Work out the finished part from the listing and answer in its coordinate system (mm). A direction names the side the tool comes from. Give positions to 0.01 mm unless a question says otherwise; leave off trailing zeros. Loops run counter-clockwise (first coordinate to the right, second up) from the corner with the lowest first, then second, coordinate; pieces in that order, holes last. Notation, with made-up numbers: (47, -0.75) - (75, -0.75) arc R29 ccw to (75, 36.25) - close; hole circle Ø9 at (-18, 12). An arc over 180 degrees is marked (long way). One line per question, with ' | ' between items.
from build123d import *

# Parameters (mm, degrees)
SKETCH2_W                = 211.751333334
SKETCH2_H                = 164
BOSS_EXTRUDE1_DEPTH      = 74.083333333
CUT_EXTRUDE7_DEPTH       = 70.90833333
CUT_EXTRUDE9_REACH       = 240.853
CUT_EXTRUDE10_DEPTH      = 3.175
SKETCH14_W               = 205.401333334
SKETCH14_H               = 3.175
CUT_EXTRUDE11_DEPTH      = 3.175
CUT_EXTRUDE12_DEPTH      = 239.853443446
CUT_EXTRUDE12_DEPTH_BACK = 3.175
CUT_EXTRUDE14_REACH      = 210.792
SKETCH18_R               = 3.025
LPATTERN2_COUNT          = 4
LPATTERN2_PITCH          = 46.99
CUT_EXTRUDE15_REACH      = 210.792
SKETCH19_R               = 3.025
LPATTERN3_COUNT          = 4
LPATTERN3_PITCH          = 46.99
BOSS_EXTRUDE2_DEPTH      = 70.866
SKETCH25_W               = 3.175
SKETCH25_H               = 19.00766667
BOSS_EXTRUDE3_DEPTH      = 3.175
CUT_EXTRUDE18_REACH      = 211.317
CUT_EXTRUDE19_REACH      = 155.042
SKETCH16_R               = 3.025
CUT_EXTRUDE20_DEPTH      = 210.317467246
LPATTERN4_COUNT          = 3
LPATTERN4_PITCH          = 50.8
SKETCH20_R               = 3.025
CUT_EXTRUDE21_DEPTH      = 210.317467246


with BuildPart() as part:
    # Sketch2 → Boss-Extrude1 (new body)
    with BuildSketch(Plane.XY):
        Rectangle(SKETCH2_W, SKETCH2_H)
    extrude(amount=BOSS_EXTRUDE1_DEPTH)

    # Sketch9 → Cut-Extrude7 (cut)
    with BuildSketch(Plane.XY.offset(74.083333333)):
        Polygon((-102.700666667, 62.95), (-102.700666667, -47.748173381), (-102.700666667, -78.825), (-61.266487403, -78.825), (102.700666667, -78.825), (102.700666667, -21.962957065), (102.700666667, 78.825), (-87.76182231, 78.825), (-102.700666667, 78.825), align=None)
    extrude(amount=-CUT_EXTRUDE7_DEPTH, mode=Mode.SUBTRACT)

    # Sketch11 → Cut-Extrude9 (cut, up to next)
    with BuildSketch(Plane.ZY.offset(105.875666667), mode=Mode.PRIVATE) as cut_extrude9_sk1:
        Polygon((58.208333333, 78.825), (74.083333333, 62.95), (74.083333333, 82), (58.208333333, 82), (58.208333333, 79.62382388), align=None)
    cut_extrude9_tool1 = extrude(cut_extrude9_sk1.sketch, amount=-CUT_EXTRUDE9_REACH, mode=Mode.PRIVATE) & part.part
    add(cut_extrude9_tool1.solids().sort_by_distance((-105.875667, 75.49881, 68.035714))[0], mode=Mode.SUBTRACT)

    # Sketch13 → Cut-Extrude10 (cut)
    with BuildSketch(Plane.ZY.offset(105.875666667)):
        Polygon((58.208333333, 78.825), (55.033333333, 82), (58.208333333, 82), align=None)
    extrude(amount=-CUT_EXTRUDE10_DEPTH, mode=Mode.SUBTRACT)

    # Sketch14 → Cut-Extrude11 (cut)
    with BuildSketch(Plane.XY.offset(58.208333333)):
        with Locations((0, 80.4125)):
            Rectangle(SKETCH14_W, SKETCH14_H)
    extrude(amount=-CUT_EXTRUDE11_DEPTH, mode=Mode.SUBTRACT)

    # Sketch15 → Cut-Extrude12 (cut, two sides: drawn at the far end of the back side and taken through both)
    with BuildSketch(Plane(origin=(105.875666667, 0, 0), x_dir=(0, 0, -1), z_dir=(1, 0, 0)).offset(-CUT_EXTRUDE12_DEPTH_BACK)):
        Polygon((-58.208333333, 79.215720039), (-58.208333333, 78.825), (-55.033333333, 82), (-58.208333333, 82), align=None)
    extrude(amount=CUT_EXTRUDE12_DEPTH + CUT_EXTRUDE12_DEPTH_BACK, mode=Mode.SUBTRACT)

    # Sketch18 → Cut-Extrude14 (cut, up to next)
    with BuildSketch(Plane.XZ.offset(82), mode=Mode.PRIVATE) as cut_extrude14_sk1:
        with Locations(Location((-89.365666667, 66.463333333, 0), (0, 0, 270))):
            Circle(SKETCH18_R)
    cut_extrude14_tool1 = extrude(cut_extrude14_sk1.sketch, amount=-CUT_EXTRUDE14_REACH, mode=Mode.PRIVATE) & part.part
    cut_extrude14 = cut_extrude14_tool1.solids().sort_by_distance((-89.365667, -82, 66.463333))[0]
    add(cut_extrude14, mode=Mode.SUBTRACT)

    # LPattern2: Cut-Extrude14 ×4
    with Locations(*[(i * LPATTERN2_PITCH, 0, 0) for i in range(1, LPATTERN2_COUNT)]):
        add(cut_extrude14, mode=Mode.SUBTRACT)

    # Sketch19 → Cut-Extrude15 (cut, up to next)
    with BuildSketch(Plane(origin=(0, 82, 0), x_dir=(1, 0, 0), z_dir=(0, 1, 0)), mode=Mode.PRIVATE) as cut_extrude15_sk1:
        with Locations(Location((-88.125666667, -48.683333333, 0), (0, 0, 270))):
            Circle(SKETCH19_R)
    cut_extrude15_tool1 = extrude(cut_extrude15_sk1.sketch, amount=-CUT_EXTRUDE15_REACH, mode=Mode.PRIVATE) & part.part
    cut_extrude15 = cut_extrude15_tool1.solids().sort_by_distance((-88.125667, 82, 48.683333))[0]
    add(cut_extrude15, mode=Mode.SUBTRACT)

    # LPattern3: Cut-Extrude15 ×4
    with Locations(*[(i * LPATTERN3_PITCH, 0, 0) for i in range(1, LPATTERN3_COUNT)]):
        add(cut_extrude15, mode=Mode.SUBTRACT)

    # Sketch22 → Boss-Extrude2 (add)
    with BuildSketch(Plane.XY.offset(3.175000003)):
        Polygon((68.717333313, 46.40313661), (68.717333313, 78.825), (71.892333313, 78.825), (71.892333313, -78.825), (68.717333313, -78.825), align=None)
    extrude(amount=BOSS_EXTRUDE2_DEPTH)

    # Sketch25 → Boss-Extrude3 (add)
    with BuildSketch(Plane(origin=(0, 78.825, 0), x_dir=(1, 0, 0), z_dir=(0, 1, 0))):
        with Locations((70.304833313, -64.537166668)):
            Rectangle(SKETCH25_W, SKETCH25_H)
    extrude(amount=BOSS_EXTRUDE3_DEPTH)

    # Sketch26 → Cut-Extrude18 (cut, up to next)
    with BuildSketch(Plane(origin=(71.892333313, 0, 0), x_dir=(0, 0, -1), z_dir=(1, 0, 0)), mode=Mode.PRIVATE) as cut_extrude18_sk1:
        Polygon((-74.083333333, 62.95), (-55.033333333, 82), (-74.041000003, 82), align=None)
    cut_extrude18_tool1 = extrude(cut_extrude18_sk1.sketch, amount=-CUT_EXTRUDE18_REACH, mode=Mode.PRIVATE) & part.part
    add(cut_extrude18_tool1.solids().sort_by_distance((71.892333, 75.65, 67.719222))[0], mode=Mode.SUBTRACT)

    # Sketch27 → Cut-Extrude19 (cut, up to next)
    with BuildSketch(Plane.XY.offset(74.083333333), mode=Mode.PRIVATE) as cut_extrude19_sk1:
        Polygon((71.892333313, -78.825), (71.892333313, -82), (105.875666667, -82), (105.875666667, 82), (71.892333313, 82), align=None)
    cut_extrude19_tool1 = extrude(cut_extrude19_sk1.sketch, amount=-CUT_EXTRUDE19_REACH, mode=Mode.PRIVATE) & part.part
    add(cut_extrude19_tool1.solids().sort_by_distance((88.884, 0, 74.083333))[0], mode=Mode.SUBTRACT)

    # Sketch16 → Cut-Extrude20 (cut, through all)
    with BuildSketch(Plane.ZY.offset(105.875666667)):
        with Locations((66.209333333, -62.95)):
            Circle(SKETCH16_R)
    cut_extrude20 = extrude(amount=-CUT_EXTRUDE20_DEPTH, mode=Mode.SUBTRACT)

    # LPattern4: Cut-Extrude20 ×3
    with Locations(*[(0, i * LPATTERN4_PITCH, 0) for i in range(1, LPATTERN4_COUNT)]):
        add(cut_extrude20, mode=Mode.SUBTRACT)

    # Sketch20 → Cut-Extrude21 (cut, through all)
    with BuildSketch(Plane.ZY.offset(105.875666667)):
        with Locations((57.72741017, 70.325667043)):
            Circle(SKETCH20_R)
    extrude(amount=-CUT_EXTRUDE21_DEPTH, mode=Mode.SUBTRACT)


solid = part.part
1. Find section A-A on y = 38.65. Write down the section's boundary in (x, z) (3 decimals).
Evaluation:
outline: (-105.876, 0) - (71.892, 0) - (71.892, 63.184) - (68.717, 63.184) - (68.717, 3.175) - (-102.701, 3.175) - (-102.701, 63.184) - (-105.876, 63.184) - close; (-105.876, 69.234) - (-102.701, 69.234) - (-102.701, 74.083) - (-105.876, 74.083) - close; (68.717, 69.234) - (71.892, 69.234) - (71.892, 74.041) - (68.717, 74.041) - close
2. Consider L1, parallel to X at y = 33.5, z = 10.5; L2, parallel to Y at x = 38.5, z = 26 (3 decimals); L3, parallel to Z at x = -3, y = 20 (3 decimals). Determine where each line is inside the solid, lowest interval first.
Evaluation:
L1: -105.88 to -102.7, 68.72 to 71.89 | L2: -82 to -78.825, 78.825 to 82 | L3: 0 to 3.175
3. Find section B-B on z = 30.5. Write down the section's boundary in (x, y) (3 decimals).
Evaluation:
outline: (-105.876, -82) - (71.892, -82) - (71.892, 82) - (-105.876, 82) - close; hole (-102.701, -78.825) - (68.717, -78.825) - (68.717, 78.825) - (-102.701, 78.825) - close
4. Find section C-C on x = -47.5. Write down the section's boundary in (y, z) (3 decimals).
Evaluation:
outline: (-82, 0) - (82, 0) - (82, 55.033) - (78.825, 55.033) - (78.825, 3.175) - (-78.825, 3.175) - (-78.825, 74.083) - (-82, 74.083) - close
5. Determine the mould class of faces 4 (the flat face through (-105.876, -1, 37)), 5 (the cylindrical face through (70.28, -9.6, 67.84)), 6 (the flat face through (-102.701, 3, 39)) for opening direction X: +X half, -X half, draft (parallel to the pull), parting line (faces both ways), or undercut.
Evaluation:
face 4: -X half | face 5: draft | face 6: undercut
6. Flat-ended cylindrical pins translate along their axes: pin 1 (1 mm diameter, centred on x = 14, y = 80, fed in from +Z); pin 2 (4 mm diameter, centred on x = -73.5, y = 22, fed in from +Z) (3 decimals); pin 3 (9.5 mm diameter, centred on x = 4.61, z = 66.46, fed in from +Y) (3 decimals). Find the tip coordinate at first contact, or state that the pin passes through.
Evaluation:
pin 1: z = 55.03 | pin 2: z = 3.175 | pin 3: y = -78.825
7. Find section D-D on y = -36. Write down the section's boundary in (x, z) (3 decimals).
Evaluation:
outline: (-105.876, 0) - (71.892, 0) - (71.892, 74.041) - (68.717, 74.041) - (68.717, 3.175) - (-102.701, 3.175) - (-102.701, 74.083) - (-105.876, 74.083) - close
8. Which of the six approach directions +Z, -Z, +X, -X, +Y, -Y give full straight-line access (tool end or side, diameter ignored) to faces 1 (the flat face through (-18, 1, 3.175)), 2 (the cylindrical face through (3.17, 80.43, 50.08)), 3 (the cylindrical face through (-39.825, -80.435, 64.837))?
Evaluation:
face 1: +Z | face 2: +Y | face 3: +Y, -Y
